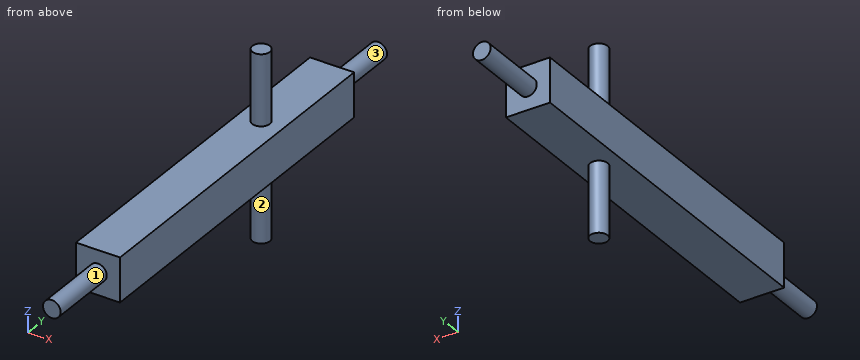
```python
from build123d import *

# Parameters (mm, degrees)
SKETCH3_W                = 25
SKETCH3_H                = 25
SKETCH3_W_2              = 22
SKETCH3_H_2              = 22
BOSS_EXTRUDE1_DEPTH      = 200
SKETCH4_R                = 5
CUT_EXTRUDE1_DEPTH       = 25
BOSS_EXTRUDE2_DEPTH      = 52.5
BOSS_EXTRUDE2_DEPTH_BACK = 52.5
SKETCH5_R                = 5
SKETCH6_W                = 25
SKETCH6_H                = 25
BOSS_EXTRUDE3_DEPTH      = 1.5
SKETCH7_W                = 25
SKETCH7_H                = 25
BOSS_EXTRUDE4_DEPTH      = 1.5
SKETCH8_R                = 5
BOSS_EXTRUDE5_DEPTH      = 40
BOSS_EXTRUDE6_START      = 40
SKETCH9_R                = 5
BOSS_EXTRUDE6_DEPTH      = 40


with BuildPart() as part:
    # Sketch3 → Boss-Extrude1 (new body)
    with BuildSketch(Plane(origin=(0, 0, 0), x_dir=(1, 0, 0), z_dir=(0, 1, 0))):
        Rectangle(SKETCH3_W, SKETCH3_H)
        Rectangle(SKETCH3_W_2, SKETCH3_H_2, mode=Mode.SUBTRACT)
    extrude(amount=BOSS_EXTRUDE1_DEPTH)

    # Sketch4 → Cut-Extrude1 (cut)
    with BuildSketch(Plane.XY.offset(12.5)):
        with Locations((0, 140)):
            Circle(SKETCH4_R)
    extrude(amount=-CUT_EXTRUDE1_DEPTH, mode=Mode.SUBTRACT)

    # Sketch5 → Boss-Extrude2 (add, two sides: drawn at the far end of the back side and taken through both)
    with BuildSketch(Plane.XY.offset(-BOSS_EXTRUDE2_DEPTH_BACK)):
        with Locations((0, 140)):
            Circle(SKETCH5_R)
    extrude(amount=BOSS_EXTRUDE2_DEPTH + BOSS_EXTRUDE2_DEPTH_BACK)

    # Sketch6 → Boss-Extrude3 (add)
    with BuildSketch(Plane(origin=(0, 200, 0), x_dir=(1, 0, 0), z_dir=(0, 1, 0))):
        Rectangle(SKETCH6_W, SKETCH6_H)
    extrude(amount=BOSS_EXTRUDE3_DEPTH)

    # Sketch7 → Boss-Extrude4 (add)
    with BuildSketch(Plane.XZ):
        Rectangle(SKETCH7_W, SKETCH7_H)
    extrude(amount=BOSS_EXTRUDE4_DEPTH)

    # Sketch8 → Boss-Extrude5 (add)
    with BuildSketch(Plane.XZ.offset(1.5)):
        with Locations(Location((0, 0, 0), (0, 0, 270))):
            Circle(SKETCH8_R)
    extrude(amount=BOSS_EXTRUDE5_DEPTH)

    # Sketch9 → Boss-Extrude6 (add)
    with BuildSketch(Plane(origin=(0, 201.5, 0), x_dir=(1, 0, 0), z_dir=(0, 1, 0)).offset(BOSS_EXTRUDE6_START)):
        with Locations(Location((0, 0, 0), (0, 0, 90))):
            Circle(SKETCH9_R)
    extrude(amount=-BOSS_EXTRUDE6_DEPTH)


solid = part.part
```
Source: CAD feature listing. Evaluate the final solid. Frame: model axes, mm. Face numbers are marked on the shaded views. A direction names the side the tool comes from. Give positions to 0.01 mm unless a question says otherwise; leave off trailing zeros. Loops run counter-clockwise (first coordinate to the right, second up) from the corner with the lowest first, then second, coordinate; pieces in that order, holes last. Notation, with made-up numbers: (43.5, 86.5) -> (56.5, 86.5) arc R14 ccw to (56.5, 101.5) -> close; hole circle Ø6 at (55.5, 23). An arc over 180 degrees is marked (long way). Use a Markdown table: item, result. Add a question column.
(1) Section query D-D (y = 80.5). Output: boundary loops of the cut face in (x, z).
(2) Section query B-B (y = 140). Output: boundary loops of the cut face in (x, z).
(3) Section query C-C (x = 0). Output: boundary loops of the cut face in (y, z), then the cut area to 4 significant figures.
(4) Section query A-A (z = 0). Output: boundary loops of the cut face in (x, y).
(5) Access query for the marked faces 1, 2 and 3. Directions: +Z, -Z, +X, -X, +Y, -Y. A direction counts if a zero-diameter tool reaches every point of the face in a straight line with its end or side. Return the directions, or none.
(6) First-contact query: pin 1 Ø4 at (x, z) = (7.5, 39) entering from +Y; pin 2 Ø6.5 at (x, y) = (-4, 72.5) entering from +Z; pin 3 Ø8 at (x, y) = (10, 62.5) entering from -Z; pin 4 Ø1.5 at (x, z) = (-2.5, -19) entering from -Y. Flat tips, straight axial feed; report the tip coordinate or a pass-through.
(7) Ray query, line 1 (Z direction, x = 7.75, y = 54.5); line 2 (Y direction, x = 2, z = -0.5); line 3 (Y direction, x = -6, z = 1). Return the intervals inside material, ascending.
Checked values:
| question | item | result |
|---|---|---|
| 1 | outline | (-12.5, -12.5) -> (12.5, -12.5) -> (12.5, 12.5) -> (-12.5, 12.5) -> close; hole (-11, -11) -> (11, -11) -> (11, 11) -> (-11, 11) -> close |
| 2 | outline | (-12.5, -12.5) -> (-5, -12.5) -> (-5, -52.5) -> (5, -52.5) -> (5, -12.5) -> (12.5, -12.5) -> (12.5, 12.5) -> (5, 12.5) -> (5, 52.5) -> (-5, 52.5) -> (-5, 12.5) -> (-12.5, 12.5) -> close; hole (-11, -11) -> (-5, -11) -> (-5, 11) -> (-11, 11) -> close; hole (5, -11) -> (11, -11) -> (11, 11) -> (5, 11) -> close |
| 3 | outline | (-41.5, -5) -> (-1.5, -5) -> (-1.5, -12.5) -> (135, -12.5) -> (135, -52.5) -> (145, -52.5) -> (145, -12.5) -> (201.5, -12.5) -> (201.5, -5) -> (241.5, -5) -> (241.5, 5) -> (201.5, 5) -> (201.5, 12.5) -> (145, 12.5) -> (145, 52.5) -> (135, 52.5) -> (135, 12.5) -> (-1.5, 12.5) -> (-1.5, 5) -> (-41.5, 5) -> close; hole (0, -11) -> (135, -11) -> (135, 11) -> (0, 11) -> close; hole (145, -11) -> (200, -11) -> (200, 11) -> (145, 11) -> close |
| 3 | area | 2,495 mm^2 |
| 4 | outline | (-12.5, -1.5) -> (-5, -1.5) -> (-5, -41.5) -> (5, -41.5) -> (5, -1.5) -> (12.5, -1.5) -> (12.5, 201.5) -> (5, 201.5) -> (5, 241.5) -> (-5, 241.5) -> (-5, 201.5) -> (-12.5, 201.5) -> close; circle Ø10 at (0, 140); hole (-11, 0) -> (11, 0) -> (11, 200) -> (-11, 200) -> close |
| 5 | face 1 | -Y |
| 5 | face 2 | -Z |
| 5 | face 3 | +Y |
| 6 | pin 1 | through |
| 6 | pin 2 | z = 12.5 |
| 6 | pin 3 | z = -12.5 |
| 6 | pin 4 | y = 135.32 |
| 7 | line 1 | -12.5 to -11, 11 to 12.5 |
| 7 | line 2 | -41.5 to 0, 135.42 to 144.58, 200 to 241.5 |
| 7 | line 3 | -1.5 to 0, 200 to 201.5 |
